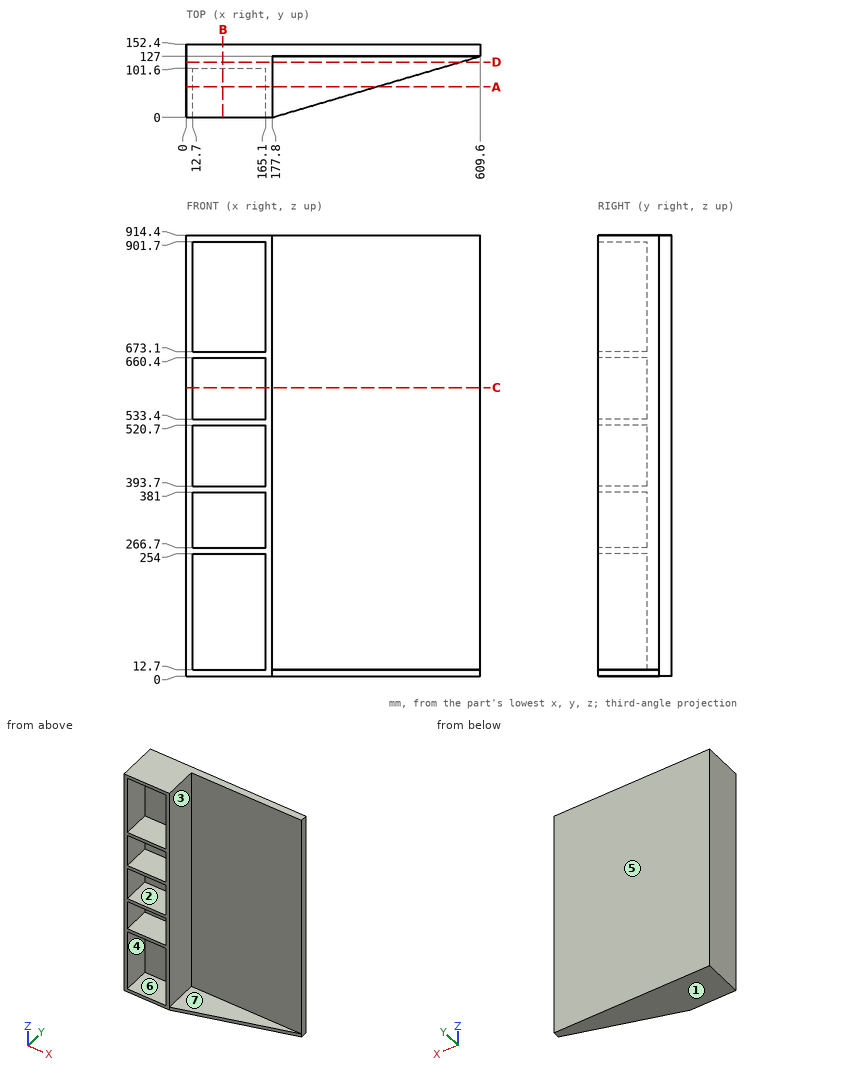
Study the drawing (mm; zero at the part's minimum x, y, z) and answer. A direction names the side the tool comes from. Coordinates: 2 decimals unless noted, no trailing zeros. Write each loop counter-clockwise with the first axis right and the second up, starting at its lowest first coordinate (ties: lowest second). Pieces come first, ordered by that corner, then holes.
Q1. A cutting plane is placed at A-A, the plane y = 63.5. Give the vertices of the cut face in (x, z).
Q2. Find the intervals of material crossed by line 1 (Z direction, x = 142.5, y = 68); line 2 (X direction, y = 30.5, z = 877.5); line 3 (Z direction, x = 562, y = 122.5), in increasing order.
Q3. Determine the mould class of the marked faces 1, 2, 3 and 4 for opening direction Z: released by +Z, released by -Z, zero draft, split by the parting line, or undercut.
Q4. A cutting plane is placed at D-D, the plane y = 115. Give the vertices of the cut face in (x, z), then the cut area to 3 significant figures.
Q5. Each of these flat-tipped pins is pushed along its axis until it touches: pin 1 Ø8 at (y, z) = (35.5, 392) entering from +X; pin 2 Ø3 at (x, z) = (421.5, 503) entering from -Y. Where does it stop, or does it pass through?
Q6. Which of the six approach directions +Z, -Z, +X, -X, +Y, -Y give full straight-line access (tool end or side, diameter ignored) to the marked faces 5, 6 and 7?
Q7. A cutting plane is placed at B-B, the plane x = 75.5. Give the vertices of the cut face in (y, z), then the cut area to 3 significant figures.
Q8. A cutting plane is placed at C-C, the plane z = 598.5. Give the vertices of the cut face in (x, y).
Findings below:
1. outline: (0, 0) - (393.7, 0) - (393.7, 12.7) - (177.8, 12.7) - (177.8, 914.4) - (0, 914.4) - close; hole (12.7, 12.7) - (165.1, 12.7) - (165.1, 254) - (12.7, 254) - close; hole (12.7, 266.7) - (165.1, 266.7) - (165.1, 381) - (12.7, 381) - close; hole (12.7, 393.7) - (165.1, 393.7) - (165.1, 520.7) - (12.7, 520.7) - close; hole (12.7, 533.4) - (165.1, 533.4) - (165.1, 660.4) - (12.7, 660.4) - close; hole (12.7, 673.1) - (165.1, 673.1) - (165.1, 901.7) - (12.7, 901.7) - close
2. line 1: z = 0 to 12.7, 254 to 266.7, 381 to 393.7, 520.7 to 533.4, 660.4 to 673.1, 901.7 to 914.4
2. line 2: x = 0 to 12.7, 165.1 to 177.8
2. line 3: z = 0 to 12.7
3. face 1: released by -Z
3. face 2: undercut
3. face 3: zero draft
3. face 4: undercut
4. outline: (0, 0) - (568.8, 0) - (568.8, 12.7) - (177.8, 12.7) - (177.8, 914.4) - (0, 914.4) - close
4. area: 168,000 mm2
5. pin 1: stops at x = 177.8
5. pin 2: stops at y = 127
6. face 5: +Z, -Z, +X, -X, +Y
6. face 6: -Y
6. face 7: +Z, +X, -Y
7. outline: (0, 0) - (152.4, 0) - (152.4, 914.4) - (0, 914.4) - (0, 901.7) - (101.6, 901.7) - (101.6, 673.1) - (0, 673.1) - (0, 660.4) - (101.6, 660.4) - (101.6, 533.4) - (0, 533.4) - (0, 520.7) - (101.6, 520.7) - (101.6, 393.7) - (0, 393.7) - (0, 381) - (101.6, 381) - (101.6, 266.7) - (0, 266.7) - (0, 254) - (101.6, 254) - (101.6, 12.7) - (0, 12.7) - close
7. area: 54,200 mm2
8. outline: (0, 0) - (12.7, 0) - (12.7, 101.6) - (165.1, 101.6) - (165.1, 0) - (177.8, 0) - (177.8, 127) - (609.6, 127) - (609.6, 152.4) - (0, 152.4) - close
